from build123d import *

# Parameters (mm, degrees)
SKETCH_1_R          = 55
SKETCH_1_R_2        = 1.5
EXTRUDE_2_DEPTH     = 3
SKETCH_2_R          = 1.5
CUT_EXTRUDE_1_DEPTH = 10


with BuildPart() as part:
    # 草图1 → 凸台-拉伸2 (new body)
    with BuildSketch(Plane(origin=(0, 0, 0), x_dir=(1, 0, 0), z_dir=(0, 1, 0))):
        with BuildLine():
            Line((-60, 70), (60, 70))
            ThreePointArc((60, 70), (130, 0), (60, -70))
            Line((60, -70), (-60, -70))
            ThreePointArc((-60, -70), (-130, 0), (-60, 70))
        make_face()
        with Locations((-60, 0)):
            Circle(SKETCH_1_R, mode=Mode.SUBTRACT)
        with Locations((60, 0)):
            Circle(SKETCH_1_R, mode=Mode.SUBTRACT)
        with Locations((-122, 0)):
            Circle(SKETCH_1_R_2, mode=Mode.SUBTRACT)
        with Locations((122, 0)):
            Circle(SKETCH_1_R_2, mode=Mode.SUBTRACT)
        with Locations((-30, 60)):
            Circle(SKETCH_1_R_2, mode=Mode.SUBTRACT)
        with Locations((30, 60)):
            Circle(SKETCH_1_R_2, mode=Mode.SUBTRACT)
        with Locations((30, -60)):
            Circle(SKETCH_1_R_2, mode=Mode.SUBTRACT)
        with Locations((-30, -60)):
            Circle(SKETCH_1_R_2, mode=Mode.SUBTRACT)
        with Locations((-49.58110934, 59.088465181)):
            Circle(SKETCH_1_R_2, mode=Mode.SUBTRACT)
        with Locations((-116.381557247, -20.5212086)):
            Circle(SKETCH_1_R_2, mode=Mode.SUBTRACT)
        with Locations((-14.037333413, -38.567256581)):
            Circle(SKETCH_1_R_2, mode=Mode.SUBTRACT)
        with Locations((14.037333413, -38.567256581)):
            Circle(SKETCH_1_R_2, mode=Mode.SUBTRACT)
        with Locations((116.381557247, -20.5212086)):
            Circle(SKETCH_1_R_2, mode=Mode.SUBTRACT)
        with Locations((49.58110934, 59.088465181)):
            Circle(SKETCH_1_R_2, mode=Mode.SUBTRACT)
    extrude(amount=EXTRUDE_2_DEPTH)

    # 草图2 → 切除-拉伸1 (cut)
    with BuildSketch(Plane(origin=(0, 3, 0), x_dir=(1, 0, 0), z_dir=(0, 1, 0))):
        with Locations((-8, -30)):
            Circle(SKETCH_2_R)
        with Locations((8, -30)):
            Circle(SKETCH_2_R)
        with Locations((8, 30)):
            Circle(SKETCH_2_R)
        with Locations((-8, 30)):
            Circle(SKETCH_2_R)
    extrude(amount=-CUT_EXTRUDE_1_DEPTH, mode=Mode.SUBTRACT)


solid = part.part
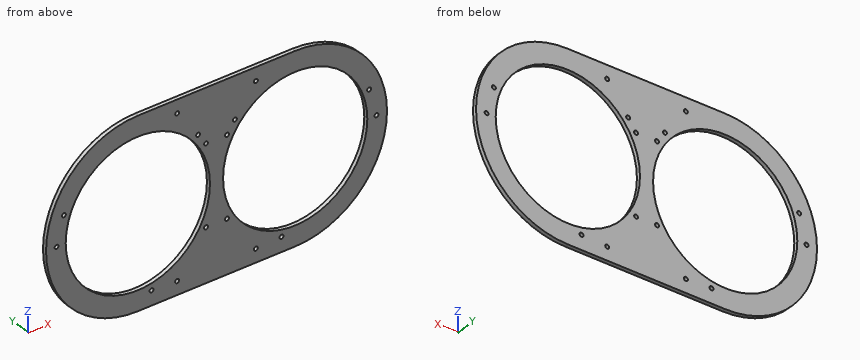
Could you check a few things on this model? Use its own coordinates, in mm. Coordinates: 2 decimals unless noted, no trailing zeros. Order: outer loops, then holes, each group sorted by start corner. A loop starts at its lowest first (then second) coordinate and runs counter-clockwise, first axis right, second up. Notation, with made-up numbers: (26.5, -29) - (65.5, -29) arc R31 ccw to (65.5, 0) - close; hole circle Ø8 at (-21.75, -1.75). An arc over 180 degrees is marked (long way). Answer in a Markdown table with one row per item. Add a question column.
(1) If we section it at C-C, the plane y = 2.25: State how many separate pieces and enclosed holes the cut face has, then the cut area to 3 significant figures.
(2) I need wall thicknesses on L1, parallel to X at y = 2.3, z = 0; L2, parallel to X at y = 2.65, z = 27; L3, parallel to Z at x = -30, y = 1.55. Which ranges of each line are inside material? Lowest first, please.
(3) Will these pins go through, and if not, where does the flat tip stop? pin 1 (2.5 mm diameter, centred on x = 122, z = 0, fed in from +Y); pin 2 (1 mm diameter, centred on x = -78.5, y = 2, fed in from +Z); pin 3 (1 mm diameter, centred on y = 0.5, z = 6, fed in from -X).
(4) If we section it at B-B, the plane x = 65.5: Please give me the cut outline in (y, z).
(5) If we section it at A-A, the plane z = 52.5: Please give me the cut outline in (x, y).
(6) If we section it at D-D, the plane z = -43: Please give me the cut outline in (x, y), then the cut area to 3 significant figures.
Results are:
| question | item | result |
|---|---|---|
| 1 | separate pieces | 1 |
| 1 | enclosed holes | 18 |
| 1 | area | 13,100 mm2 |
| 2 | L1 | x = -130 to -123.5, -120.5 to -115, -5 to 5, 115 to 120.5, 123.5 to 130 |
| 2 | L2 | x = -124.58 to -107.92, -12.08 to 12.08, 107.92 to 124.58 |
| 2 | L3 | z = -70 to -61.5, -58.5 to -46.1, 46.1 to 58.5, 61.5 to 70 |
| 3 | pin 1 | passes through |
| 3 | pin 2 | stops at z = 67.65 |
| 3 | pin 3 | stops at x = -129.78 |
| 4 | outline | (0, -69.78) - (3, -69.78) - (3, -54.72) - (0, -54.72) - close; (0, 54.72) - (3, 54.72) - (3, 69.78) - (0, 69.78) - close |
| 5 | outline | (-106.3, 0) - (-76.39, 0) - (-76.39, 3) - (-106.3, 3) - close; (-43.61, 0) - (43.61, 0) - (43.61, 3) - (-43.61, 3) - close; (76.39, 0) - (106.3, 0) - (106.3, 3) - (76.39, 3) - close |
| 6 | outline | (-115.24, 0) - (-94.29, 0) - (-94.29, 3) - (-115.24, 3) - close; (-25.71, 0) - (25.71, 0) - (25.71, 3) - (-25.71, 3) - close; (94.29, 0) - (115.24, 0) - (115.24, 3) - (94.29, 3) - close |
| 6 | area | 280 mm2 |
